from build123d import *

# Parameters (mm, degrees)
F0_R     = 38
F0_R_2   = 21.5
F1_DEPTH = 10
F3_DEPTH = 10
F4_DEPTH = 5


with BuildPart() as f1:
    # F0 (on Top) → F1 (new body)
    with BuildSketch(Plane.XY):
        Circle(F0_R)
        Circle(F0_R_2, mode=Mode.SUBTRACT)
    extrude(amount=F1_DEPTH)

    # F2 (on face) → F3 (cut)
    with BuildSketch(Plane.XY.offset(10)):
        with BuildLine():
            ThreePointArc((17.3950694854, 25.5037771635), (18.7013512829, 23.576948176), (20.9465824354, 24.1917482683))
            ThreePointArc((20.9465824354, 24.1917482683), (19.3944253287, 25.4530207671), (17.7665087481, 26.6148674035))
            ThreePointArc((17.7665087481, 26.6148674035), (17.4976104485, 26.0871290467), (17.3950694854, 25.5037771635))
        make_face()
        with BuildLine():
            ThreePointArc((17.7665087481, 26.6148674035), (19.3944253287, 25.4530207671), (20.9465824354, 24.1917482683))
            ThreePointArc((20.9465824354, 24.1917482683), (21.2791420466, 24.7838101177), (21.3944253287, 25.4530207671))
            ThreePointArc((21.3944253287, 25.4530207671), (20.0044117379, 27.3577298212), (17.7665087481, 26.6148674035))
        make_face()
        with BuildLine():
            ThreePointArc((33.4880347509, -5.7011987796), (33.0028452429, -4.3953085953), (31.7826855775, -3.7230226271))
            ThreePointArc((31.7826855775, -3.7230226271), (31.6508184403, -4.7144132252), (31.4880347509, -5.7011987796))
            ThreePointArc((31.4880347509, -5.7011987796), (31.2944935166, -6.6824153971), (31.0703837886, -7.6571046244))
            ThreePointArc((31.0703837886, -7.6571046244), (32.7459493099, -7.2560785056), (33.4880347509, -5.7011987796))
        make_face()
        with BuildLine():
            ThreePointArc((31.4880347509, -5.7011987796), (31.6508184403, -4.7144132252), (31.7826855775, -3.7230226271))
            ThreePointArc((31.7826855775, -3.7230226271), (29.7436669076, -4.7228425934), (29.9536778777, -6.9840662652))
            Line((29.9536778777, -6.9840662652), (31.4880347509, -5.7011987796))
        make_face()
        with BuildLine():
            ThreePointArc((31.0703837886, -7.6571046244), (31.2944935166, -6.6824153971), (31.4880347509, -5.7011987796))
            Line((31.4880347509, -5.7011987796), (29.9536778777, -6.9840662652))
            ThreePointArc((29.9536778777, -6.9840662652), (30.4556448993, -7.414141042), (31.0703837886, -7.6571046244))
        make_face()
        with BuildLine():
            ThreePointArc((-17.3276317844, 25.5037771635), (-17.4221248046, 26.1112663816), (-17.6966749345, 26.6613521087))
            ThreePointArc((-17.6966749345, 26.6613521087), (-19.3276317844, 25.5037771635), (-20.8830900727, 24.2465780888))
            ThreePointArc((-20.8830900727, 24.2465780888), (-18.6608921713, 23.6181848724), (-17.3276317844, 25.5037771635))
        make_face()
        with BuildLine():
            ThreePointArc((-20.8830900727, 24.2465780888), (-19.3276317844, 25.5037771635), (-17.6966749345, 26.6613521087))
            ThreePointArc((-17.6966749345, 26.6613521087), (-20.5356087709, 27.0977632362), (-20.8830900727, 24.2465780888))
        make_face()
        with BuildLine():
            Line((0.0337188505, -31.999982235), (1.5680757237, -30.7171147494))
            ThreePointArc((1.5680757237, -30.7171147494), (0.8805556201, -30.1881137283), (0.0337188505, -29.999982235))
            Line((0.0337188505, -29.999982235), (0.0337188505, -31.999982235))
        make_face()
        with BuildLine():
            ThreePointArc((2.0326750825, -31.9353758708), (1.9024391118, -31.2873220179), (1.5680757237, -30.7171147494))
            Line((1.5680757237, -30.7171147494), (0.0337188505, -31.999982235))
            ThreePointArc((0.0337188505, -31.999982235), (1.033701827, -31.983299713), (2.0326750825, -31.9353758708))
        make_face()
        with BuildLine():
            ThreePointArc((2.0337188505, -31.999982235), (2.0334578915, -31.9676748374), (2.0326750825, -31.9353758708))
            ThreePointArc((2.0326750825, -31.9353758708), (1.033701827, -31.983299713), (0.0337188505, -31.999982235))
            ThreePointArc((0.0337188505, -31.999982235), (-0.9662970627, -31.9854071412), (-1.9653690958, -31.9395886686))
            ThreePointArc((-1.9653690958, -31.9395886686), (0.003518624, -33.9997542086), (2.0337188505, -31.999982235))
        make_face()
        with BuildLine():
            Line((0.0337188505, -31.999982235), (0.0337188505, -29.999982235))
            ThreePointArc((0.0337188505, -29.999982235), (-0.8150266404, -30.189007058), (-1.503338165, -30.7203511432))
            Line((-1.503338165, -30.7203511432), (0.0337188505, -31.999982235))
        make_face()
        with BuildLine():
            ThreePointArc((-1.9653690958, -31.9395886686), (-0.9662970627, -31.9854071412), (0.0337188505, -31.999982235))
            Line((0.0337188505, -31.999982235), (-1.503338165, -30.7203511432))
            ThreePointArc((-1.503338165, -30.7203511432), (-1.8364991405, -31.2912617919), (-1.9653690958, -31.9395886686))
        make_face()
        with BuildLine():
            ThreePointArc((-29.4759499676, -5.7675448535), (-30.1716566854, -4.2513591676), (-31.7747690017, -3.7899940488))
            ThreePointArc((-31.7747690017, -3.7899940488), (-31.640812874, -4.7811045451), (-31.4759499676, -5.7675448535))
            Line((-31.4759499676, -5.7675448535), (-29.9388929521, -7.0471759453))
            ThreePointArc((-29.9388929521, -7.0471759453), (-29.5952434473, -6.4479439896), (-29.4759499676, -5.7675448535))
        make_face()
        with BuildLine():
            ThreePointArc((-31.4759499676, -5.7675448535), (-31.640812874, -4.7811045451), (-31.7747690017, -3.7899940488))
            ThreePointArc((-31.7747690017, -3.7899940488), (-33.4431968406, -6.1280164068), (-31.054178004, -7.722566186))
            ThreePointArc((-31.054178004, -7.722566186), (-31.2803413207, -6.7483514181), (-31.4759499676, -5.7675448535))
        make_face()
        with BuildLine():
            Line((-29.9388929521, -7.0471759453), (-31.4759499676, -5.7675448535))
            ThreePointArc((-31.4759499676, -5.7675448535), (-31.2803413207, -6.7483514181), (-31.054178004, -7.722566186))
            ThreePointArc((-31.054178004, -7.722566186), (-30.4399525078, -7.4783076258), (-29.9388929521, -7.0471759453))
        make_face()
    extrude(amount=-F3_DEPTH, mode=Mode.SUBTRACT)

    # F4 (add): a face of the model
    f4_faces = [f1.faces().sort_by_distance(p)[0] for p in [
        (-36.9251976926, 0, 10),
    ]]
    extrude(f4_faces, amount=F4_DEPTH)


solid = f1.part
CAD build for the part. Positions are in the model's coordinates, mm. Round coordinates to 2 decimals unless told otherwise and drop trailing zeros. Write each loop counter-clockwise with the first axis right and the second up, starting at its lowest first coordinate (ties: lowest second). Pieces come first, ordered by that corner, then holes.
(1) Slice it at B-B, the plane z = 6.5. Write the cut outline in (x, y), and give its area (3 significant figures).
(2) Drop flat-ended pins along their axis: P1, Ø3, axis at x = -2, y = -19, coming from the +Z side; P2, Ø8, axis at x = -17, z = 12.5, coming from the +Y side; P3, Ø4, axis at y = -3.5, z = 3, coming from the +X side; P4, Ø2, axis at y = -26.5, z = 3, coming from the -X side. Give the stop position or say it passes through.
(3) Slice it at C-C, the plane x = 10. Write the cut outline in (y, z), and give its area (3 significant figures).
(4) Probe line 1 along Y through (x, z) = (0, 4.5); line 2 along X through (y, z) = (-4.5, 2.75); line 3 along Y through (x, z) = (14, 11). List the from-to ranges inside material, lowest first.
(5) Slice it at A-A, the plane y = 0. Write the cut outline in (x, z).
(6) Slice it at D-D, the plane y = 31. Write the cut outline in (x, z), and give its area (3 significant figures).
From the geometry:
1. outline: circle Ø76 at (0, 0); hole circle Ø4 at (-31.48, -5.77); hole circle Ø43 at (0, 0); hole circle Ø4 at (-19.33, 25.5); hole circle Ø4 at (0.03, -32); hole circle Ø4 at (19.39, 25.45); hole circle Ø4 at (31.49, -5.7)
1. area: 3,020 mm2
2. P1: passes through
2. P2: stops at y = 35.71
2. P3: stops at x = 37.97
2. P4: stops at x = -28.17
3. outline: (-36.66, 0) - (-19.03, 0) - (-19.03, 15) - (-36.66, 15) - close; (19.03, 0) - (36.66, 0) - (36.66, 15) - (19.03, 15) - close
3. area: 529 mm2
4. line 1: y = -38 to -34, -30 to -21.5, 21.5 to 38
4. line 2: x = -37.73 to -33.02, -29.93 to -21.02, 21.02 to 29.89, 33.09 to 37.73
4. line 3: y = -35.33 to -16.32, 16.32 to 35.33
5. outline: (-38, 0) - (-21.5, 0) - (-21.5, 15) - (-38, 15) - close; (21.5, 0) - (38, 0) - (38, 15) - (21.5, 15) - close
6. outline: (-21.98, 0) - (21.98, 0) - (21.98, 15) - (-21.98, 15) - close
6. area: 659 mm2
